Work out the finished part from the listing and answer in its coordinate system (mm). Face numbers are marked on the shaded views. A direction names the side the tool comes from. Round coordinates to 2 decimals unless told otherwise and drop trailing zeros. Loops run counter-clockwise (first coordinate to the right, second up) from the corner with the lowest first, then second, coordinate; pieces in that order, holes last. Notation, with made-up numbers: (76.25, 6) - (98.25, 6) arc R29 ccw to (98.25, 45) - close; hole circle Ø1 at (-10.75, 71). An arc over 180 degrees is marked (long way). Answer as CSV lines item,"result". Start each with the question number.
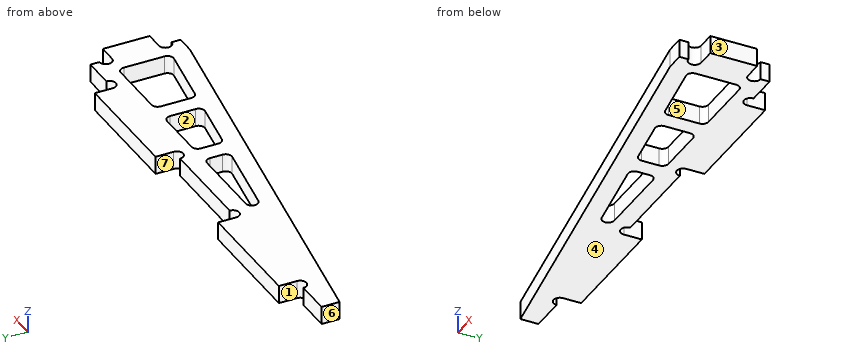
```python
from build123d import *

# Parameters (mm, degrees)
EXTRUDE_1_DEPTH = 3
FILLET_1_R      = 1.01


with BuildPart() as part:
    # 草图1 → 凸台-拉伸1 (new body)
    with BuildSketch(Plane.XY):
        with BuildLine():
            Line((-11.95, -1.5), (-28.05, -1.5))
            ThreePointArc((-28.05, -1.5), (-29.1, -2.55), (-30.15, -1.5))
            Line((-30.15, -1.5), (-30.15, 1.5))
            Line((-30.15, 1.5), (-49.85, 1.5))
            Line((-49.85, 1.5), (-49.85, -1.5))
            ThreePointArc((-49.85, -1.5), (-50.9, -2.55), (-51.95, -1.5))
            Line((-51.95, -1.5), (-57.85, -1.5))
            Line((-57.85, -1.5), (-57.85, -4.5))
            Line((-57.85, -4.5), (14.15, -16.5))
            Line((14.15, -16.5), (17.15, -16.5))
            Line((17.15, -16.5), (17.15, -15))
            ThreePointArc((17.15, -15), (16.1, -13.95), (17.15, -12.9))
            Line((17.15, -12.9), (20.15, -12.9))
            Line((20.15, -12.9), (20.15, -5.1))
            Line((20.15, -5.1), (17.15, -5.1))
            ThreePointArc((17.15, -5.1), (16.1, -4.05), (17.15, -3))
            Line((17.15, -3), (17.15, -1.5))
            Line((17.15, -1.5), (11.95, -1.5))
            ThreePointArc((11.95, -1.5), (10.9, -2.55), (9.85, -1.5))
            Line((9.85, -1.5), (9.85, 1.5))
            Line((9.85, 1.5), (-9.85, 1.5))
            Line((-9.85, 1.5), (-9.85, -1.5))
            ThreePointArc((-9.85, -1.5), (-10.9, -2.55), (-11.95, -1.5))
        make_face()
        Polygon((-10.85, -9.291952068), (-10.85, -4.5), (-0.85, -4.5), (-0.85, -10.958618735), align=None, mode=Mode.SUBTRACT)
        Polygon((2.15, -4.5), (14.15, -4.5), (14.15, -13.458618735), (2.15, -11.458618735), align=None, mode=Mode.SUBTRACT)
        Polygon((-13.85, -8.791952068), (-39.601712409, -4.5), (-13.85, -4.5), align=None, mode=Mode.SUBTRACT)
    extrude(amount=EXTRUDE_1_DEPTH)

    # 圆角1
    fillet_1_edges = [part.edges().sort_by_distance(p)[0] for p in [
        (-0.85, -4.5, 1.5),
        (-10.85, -4.5, 1.5),
        (-10.85, -9.291952068, 1.5),
        (-0.85, -10.958618735, 1.5),
        (2.15, -11.458618735, 1.5),
        (14.15, -13.458618735, 1.5),
        (14.15, -4.5, 1.5),
        (2.15, -4.5, 1.5),
        (-13.85, -4.5, 1.5),
        (-39.601712409, -4.5, 1.5),
        (-13.85, -8.791952068, 1.5),
    ]]
    fillet(fillet_1_edges, radius=FILLET_1_R)


solid = part.part
```
Item 1: Which of the six approach directions +Z, -Z, +X, -X, +Y, -Y give full straight-line access (tool end or side, diameter ignored) to the marked faces 5, 6 and 7?
Item 2: Section C-C, the plane x = -18.5 is taken. Give the vertices of the cut face in (y, z), and give its area (3 significant figures).
Item 3: Section B-B, the plane z = 1.45 is taken. Count the separate pieces of the cut face and the enclosed holes in it, and give its area (3 significant figures).
Item 4: Section D-D, the plane x = -49 is taken. Give the vertices of the cut face in (y, z) (3 decimals), and give its area (3 significant figures).
Item 5: Determine the mould class of the marked faces 1, 2, 3 and 4 for opening direction X: pulls with the +X half, pulls with the -X half, needs draft (parallel to the pull), parting line crosses it, or undercut.
Item 6: Section A-A, the plane x = 4 is taken. Give the vertices of the cut face in (y, z), and give its area (3 significant figures).
Item 7: Flat-ended cylindrical pins translate along their axes: pin 1 Ø0.8 at (y, z) = (-16, 1) entering from +X; pin 2 Ø0.9 at (x, z) = (-53.5, 1) entering from +Y; pin 3 Ø0.9 at (x, z) = (-23, 2) entering from -Y. Find the tip coordinate at first contact, or state that the pin passes through.
Item 8: Find the intervals of material crossed by L1, parallel to X at y = -0.25, z = 2.95; L2, parallel to Y at x = -25, z = 2.8 (3 decimals); L3, parallel to Y at x = -10.5, z = 1.7, in increasing order.
Answer:
1,face 5,"+Z, -Z"
1,face 6,"+Z, -Z, -X, +Y, -Y"
1,face 7,"+Z, -Z, +Y"
2,outline,"(-11.06, 0) - (-8.02, 0) - (-8.02, 3) - (-11.06, 3) - close; (-4.5, 0) - (-1.5, 0) - (-1.5, 3) - (-4.5, 3) - close"
2,area,"18.1 mm²"
3,separate pieces,"1"
3,enclosed holes,"3"
3,area,"630 mm²"
4,outline,"(-5.975, 0) - (1.5, 0) - (1.5, 3) - (-5.975, 3) - close"
4,area,"22.4 mm²"
5,face 1,"pulls with the -X half"
5,face 2,"undercut"
5,face 3,"pulls with the +X half"
5,face 4,"needs draft"
6,outline,"(-14.81, 0) - (-11.77, 0) - (-11.77, 3) - (-14.81, 3) - close; (-4.5, 0) - (1.5, 0) - (1.5, 3) - (-4.5, 3) - close"
6,area,"27.1 mm²"
7,pin 1,"stops at x = 17.15"
7,pin 2,"stops at y = -1.5"
7,pin 3,"stops at y = -10.38"
8,L1,"x = -49.85 to -30.15, -9.85 to 9.85"
8,L2,"y = -9.975 to -6.934, -4.5 to -1.5"
8,L3,"y = -12.39 to -9.2, -4.75 to -2.47"
